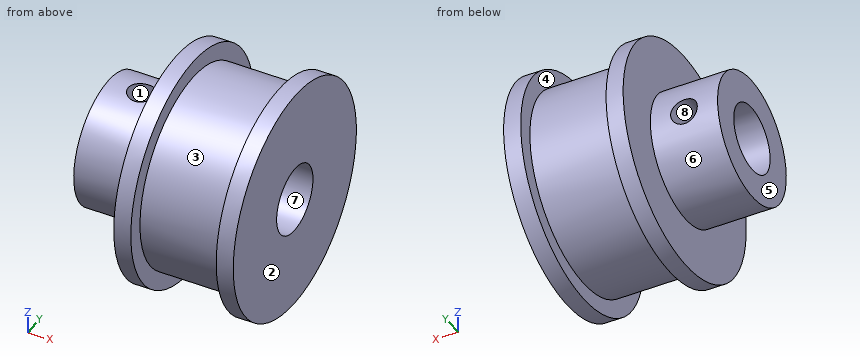
from build123d import *

# Parameters (mm, degrees)
SKETCH2_R                       = 6
BOSS_EXTRUDE1_DEPTH             = 6.3
HOLE1_D                         = 6.35
SKETCH5_W                       = 1.25
SKETCH5_H                       = 7.831417296
F_2_5_2_5_DIAMETER_HOLE2_REACH  = 26.537
F_2_5_2_5_DIAMETER_HOLE2_BORE_R = 1.25


with BuildPart() as part:
    # Sketch1 → Revolve1 (revolve)
    with BuildSketch(Plane.XY, mode=Mode.PRIVATE) as revolve1_sk:
        Polygon((6.3, 10.75), (6.3, 0), (17.5, 0), (17.5, 10.75), (15.9, 10.75), (15.9, 9.15), (7.9, 9.15), (7.9, 10.75), align=None)
    revolve(revolve1_sk.sketch.rotate(Axis((6.3, 0, 0), (1, 0, 0)), 270), axis=Axis((6.3, 0, 0), (1, 0, 0)))

    # Sketch2 → Boss-Extrude1 (add)
    with BuildSketch(Plane.ZY.offset(-6.3)):
        Circle(SKETCH2_R)
    extrude(amount=BOSS_EXTRUDE1_DEPTH)

    # Hole1 (through all)
    with Locations(Plane.ZY):
        with Locations((0, 0)):
            Hole(HOLE1_D / 2)

    # Sketch5 → Ø2.5 (2.5) Diameter Hole1 (revolve, cut)
    with BuildSketch(Plane(origin=(3.15, 2.918582704, 0), x_dir=(0, 0, -1), z_dir=(1, 0, 0))):
        with Locations((0.625, 3.915708648)):
            Rectangle(SKETCH5_W, SKETCH5_H)
    revolve(axis=Axis((3.15, -3.431417296, 0), (0, 1, 0)), mode=Mode.SUBTRACT)

    # Ø2.5 (2.5) Diameter Hole2 bore (on position points) → Ø2.5 (2.5) Diameter Hole2 (cut, up to next)
    with BuildSketch(Plane(origin=(3.15, 0, 6), x_dir=(0, 1, 0), z_dir=(0, 0, 1)), mode=Mode.PRIVATE) as f_2_5_2_5_diameter_hole2_sk1:
        Circle(F_2_5_2_5_DIAMETER_HOLE2_BORE_R)
    f_2_5_2_5_diameter_hole2_tool1 = extrude(f_2_5_2_5_diameter_hole2_sk1.sketch, amount=-F_2_5_2_5_DIAMETER_HOLE2_REACH, mode=Mode.PRIVATE) & part.part
    add(f_2_5_2_5_diameter_hole2_tool1.solids().sort_by_distance((3.15, 0, 6))[0], mode=Mode.SUBTRACT)


solid = part.part
CAD build for the part. Positions are in the model's coordinates, mm. Face numbers are marked on the shaded views. A direction names the side the tool comes from. Round coordinates to 2 decimals unless told otherwise and drop trailing zeros. Order: outer loops, then holes, each group sorted by start corner. A loop starts at its lowest first (then second) coordinate and runs counter-clockwise, first axis right, second up. Notation, with made-up numbers: M -37,52 L 14,52 A31 cw 14,76 Z; hole C 48.25,-19.75 d5. An arc over 180 degrees is marked long. Use one line per item in the form item = value.
Q1. Two-plate mould, pull along Y, no slides. Class the marked faces 1, 2 and 3: +Y half, -Y half, draft (parallel to the pull), parting line (faces both ways), or undercut.
Recorded:
face_1 = undercut
face_2 = draft
face_3 = parting line
Q2. Probe L1, parallel to Y at x = 6.25, z = 0 (3 decimals); L2, parallel to X at y = 4, z = 0; L3, parallel to X at y = -10, z = -2.75. List the from-to ranges inside material, lowest first.
Recorded:
L1 = -6 to -3.175, 3.175 to 6
L2 = 0 to 1.9, 4.4 to 17.5
L3 = 6.3 to 7.9, 15.9 to 17.5
Q3. Saw through at D-D on x = 3.15. Give the cut face in (y, z) (3 decimals), then the cut area to 3 significant figures.
Recorded:
outline = M -1.25,2.919 L -1.25,5.868 A6 ccw long 5.868,-1.25 L 2.919,-1.25 A3.175 cw long Z; M 1.25,2.919 A3.175 cw 2.919,1.25 L 5.868,1.25 A6 ccw 1.25,5.868 Z
area = 67.1 mm^2
Q4. Saw through at A-A on z = 0. Give the cut face in (x, y) (3 decimals).
Recorded:
outline = M 0,-6 L 6.3,-6 L 6.3,-10.75 L 7.9,-10.75 L 7.9,-9.15 L 15.9,-9.15 L 15.9,-10.75 L 17.5,-10.75 L 17.5,-3.175 L 0,-3.175 Z; M 0,3.175 L 1.9,3.175 L 1.9,6 L 0,6 Z; M 4.4,3.175 L 17.5,3.175 L 17.5,10.75 L 15.9,10.75 L 15.9,9.15 L 7.9,9.15 L 7.9,10.75 L 6.3,10.75 L 6.3,6 L 4.4,6 Z
Q5. Saw through at C-C on z = 2.25. Give the cut face in (x, y).
Recorded:
outline = M 0,-5.56 L 6.3,-5.56 L 6.3,-10.51 L 7.9,-10.51 L 7.9,-8.87 L 15.9,-8.87 L 15.9,-10.51 L 17.5,-10.51 L 17.5,-2.24 L 0,-2.24 Z; M 0,2.24 L 17.5,2.24 L 17.5,10.51 L 15.9,10.51 L 15.9,8.87 L 7.9,8.87 L 7.9,10.51 L 6.3,10.51 L 6.3,5.56 L 0,5.56 Z
Q6. Which spindle directions (+Z, -Z, +X, -X, +Y, -Y) get a long thin tool onto all of the face, cutting with end or side? Do the marked faces 4, 5, 6, 7 and 8. Say none if no direction does.
Recorded:
face_4 = none
face_5 = +Z, -Z, -X, +Y, -Y
face_6 = -X
face_7 = +X, -X
face_8 = +Y
Q7. Flat gauge pins, fed straight in: P1, Ø4, axis at y = 0, z = 0, coming from the -X side; P2, Ø4, axis at x = 14, z = 4, coming from the +Y side; P3, Ø3, axis at x = 4.5, y = 7, coming from the -Z side; P4, Ø1.5, axis at x = 11, z = 3.5, coming from the +Y side. Where does each tip first touch, or does it go through?
Recorded:
P1 = through
P2 = 10.21
P3 = -2.4
P4 = 8.73
